Could you check a few things on this model? Use its own coordinates, in mm. Face numbers are marked on the shaded views. Give positions to 0.01 mm unless a question says otherwise; leave off trailing zeros. Order: outer loops, then holes, each group sorted by start corner. A loop starts at its lowest first (then second) coordinate and runs counter-clockwise, first axis right, second up. Notation, with made-up numbers: (33.5, 7) - (44.5, 7) arc R20 ccw to (44.5, 43) - close; hole circle Ø9 at (58.25, 19). An arc over 180 degrees is marked (long way). One line per question, with ' | ' between items. Start each with the question number.
1. Imagine slicing it at A-A (y = 0). Please give me the cut outline in (x, z), and give its area (3 significant figures).
2. Imagine slicing it at C-C (x = 11.5). Please give me the cut outline in (y, z).
3. For P1, Ø1, axis at x = 12.5, z = -0.5, coming from the +Y side; P2, Ø1.5, axis at x = 8, z = -0.5, coming from the -Y side, each with a flat end and sliding along its axis, tell me the tip position at first contact or that it passes through.
4. Imagine slicing it at D-D (x = -0.5). Please give me the cut outline in (y, z), and give its area (3 significant figures).
5. If we mould it in two halves opening along X, with no side actions, what happens to the marked faces 1, 2 and 3? For each: released by +X, released by -X, zero draft, split by the parting line, or undercut.
6. I need wall thicknesses on probe 1 along Y at (x, z) = (18.75, 0.15); probe 2 along Y at (x, z) = (5.5, 1.5). Which ranges of each line are inside material? Lowest first, please. Write a range as from..to.
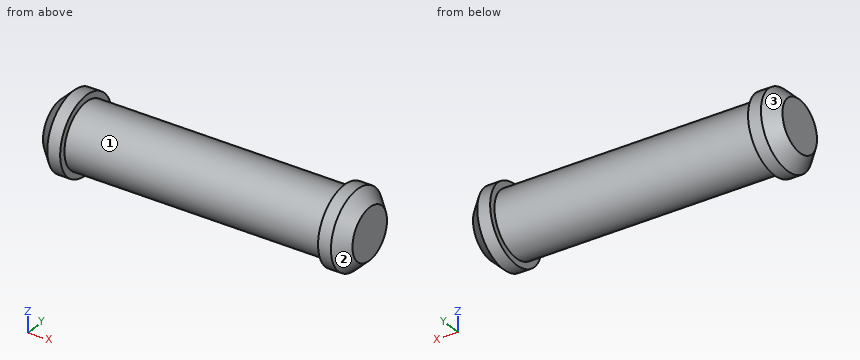
Autodesk Inventor part; units mm, degrees
ref_plane "YZ Plane" through (0, 0, 0) normal (1, 0, 0) x (0, 1, 0)
ref_plane "XZ Plane" through (0, 0, 0) normal (0, 1, 0) x (-1, 0, 0)
ref_plane "XY Plane" through (0, 0, 0) normal (0, 0, 1) x (1, 0, 0)
sketch "Sketch1" plane through (0, 0, 0) normal (1, 0, 0) x (0, 1, 0)
  circle A0 centre (0, 0) radius 2.5
  dimension "d0" = 5
extrude "Extrusion1" add sketch "Sketch1" along normal blind 20
sketch "Sketch2" plane through (20, 0, 0) normal (1, 0, 0) x (0, 0, -1)
  circle A0 centre (0, 0) radius 3
  dimension "d3" = 6
extrude "Extrusion2" add sketch "Sketch2" along normal blind 2
chamfer "Chamfer1" distance 1 angle 45 1 edges at (22, 0, 3)
sketch "Sketch3" plane through (0, 0, 0) normal (-1, 0, 0) x (0, 0, 1)
  circle A0 centre (0, 0) radius 3
extrude "Extrusion3" add sketch "Sketch3" along normal blind 2
chamfer "Chamfer2" distance 1 angle 45 1 edges at (-2, 0, -3)
properties part number "Shaft"
Results found:
1) outline: (-2, -2) - (-1, -3) - (0, -3) - (0, -2.5) - (20, -2.5) - (20, -3) - (21, -3) - (22, -2) - (22, 2) - (21, 3) - (20, 3) - (20, 2.5) - (0, 2.5) - (0, 3) - (-1, 3) - (-2, 2) - close | area: 122 mm2
2) outline: circle Ø5 at (0, 0)
3) P1: stops at y = 2.5 | P2: stops at y = -2.5
4) outline: circle Ø6 at (0, 0) | area: 28.3 mm2
5) face 1: undercut | face 2: released by +X | face 3: released by -X
6) probe 1: y = -2.5..2.5 | probe 2: y = -2..2
